Here's how the part is built. I have some questions about the finished solid (model axes, mm). Face numbers are marked on the shaded views. A direction names the side the tool comes from. Coordinates: 2 decimals unless noted, no trailing zeros. Write each loop counter-clockwise with the first axis right and the second up, starting at its lowest first coordinate (ties: lowest second). Pieces come first, ordered by that corner, then holes.
(1) Imagine slicing it at B-B, the plane x = 0. List the corners of the cut face in (y, z) for me, plus the area to 3 significant figures.
(2) Imagine slicing it at A-A, the plane y = 15.3. List the corners of the cut face in (x, z) for me.
(3) For pin 1 Ø1.5 at (x, y) = (39.99, 15.3) entering from -Z; pin 2 Ø3.5 at (x, y) = (34.5, -16) entering from +Z; pin 3 Ø1.6 at (y, z) = (12, -101.5) entering from -X; pin 4 Ø2.5 at (y, z) = (-16, -100.5) entering from -X, each with a flat end and sliding along its axis, tell me the tip position at first contact or that it passes through.
(4) Imagine slicing it at C-C, the plane x = 32. List the corners of the cut face in (y, z) for me, plus the area to 3 significant figures.
(5) Which directions (+Z, -Z, +X, -X, +Y, -Y) give clear straight access to the entire face, cutting with the end or side of a thin tool? Please do the marked faces 1, 2 and 3.
(6) Please list where these lines run through material, in increasing order: probe 1 along Y at (x, z) = (16, -88.25); probe 2 along Z at (x, y) = (38.5, -15.5); probe 3 along Z at (x, y) = (42, 12.5).
(7) Imagine slicing it at D-D, the plane y = -8. List the corners of the cut face in (x, z) for me, plus the area to 3 significant figures.
```python
from build123d import *

# Parameters (mm, degrees)
SKETCH_1_R          = 1.6
EXTRUDE_1_DEPTH     = 3
SKETCH_2_R          = 3.1
CUT_EXTRUDE_1_DEPTH = 2
FILLET_1_R          = 0.2
SKETCH_4_W          = 20
SKETCH_4_H          = 3.3
EXTRUDE_2_DEPTH     = 37
FILLET_2_R          = 2
SKETCH_5_R          = 1.25
CUT_EXTRUDE_2_DEPTH = 3.3


with BuildPart() as part:
    # Эскиз1 → Бобышка-Вытянуть1 (new body)
    with BuildSketch(Plane(origin=(0, -18, 0), x_dir=(1, 0, 0), z_dir=(0, 1, 0))):
        with BuildLine():
            Line((9.520833333, 86.731463811), (-1.458333333, 90.079283893))
            ThreePointArc((-1.458333333, 90.079283893), (-5, 94.861884011), (-1.458333333, 99.644484129))
            Line((-1.458333333, 99.644484129), (6.608333333, 102.104210763))
            ThreePointArc((6.608333333, 102.104210763), (7.495119036, 101.951328303), (7.9, 101.14769074))
            Line((7.9, 101.14769074), (7.9, 94.861884011))
            ThreePointArc((7.9, 94.861884011), (12, 90.761884011), (16.1, 94.861884011))
            Line((16.1, 94.861884011), (16.1, 102.361884011))
            ThreePointArc((16.1, 102.361884011), (16.392893219, 103.068990793), (17.1, 103.361884011))
            Line((17.1, 103.361884011), (44.988630488, 103.361884011))
            Line((44.988630488, 103.361884011), (44.988630488, 94.861884011))
            Line((44.988630488, 94.861884011), (29, 94.861884011))
            ThreePointArc((29, 94.861884011), (28.018187817, 91.886288833), (25.458333333, 90.079283893))
            Line((25.458333333, 90.079283893), (14.479166667, 86.731463811))
            ThreePointArc((14.479166667, 86.731463811), (12, 86.361884011), (9.520833333, 86.731463811))
        make_face()
        with Locations(Location((24, 94.861884011, 0), (0, 0, 270))):
            Circle(SKETCH_1_R, mode=Mode.SUBTRACT)
        with Locations(Location((0, 94.861884011, 0), (0, 0, 270))):
            Circle(SKETCH_1_R, mode=Mode.SUBTRACT)
    extrude(amount=EXTRUDE_1_DEPTH)

    # Эскиз2 → Вырез-Вытянуть1 (cut)
    with BuildSketch(Plane(origin=(0, -15, 0), x_dir=(1, 0, 0), z_dir=(0, 1, 0))):
        with Locations(Location((0, 94.861884011, 0), (0, 0, 270))):
            Circle(SKETCH_2_R)
        with Locations(Location((24, 94.861884011, 0), (0, 0, 270))):
            Circle(SKETCH_2_R)
    extrude(amount=-CUT_EXTRUDE_1_DEPTH, mode=Mode.SUBTRACT)

    # Скругление1
    fillet_1_edges = [part.edges().sort_by_distance(p)[0] for p in [
        (0, -17, -97.961884011),
        (24, -17, -97.961884011),
    ]]
    fillet(fillet_1_edges, radius=FILLET_1_R)

    # Эскиз4 → Бобышка-Вытянуть2 (add)
    with BuildSketch(Plane(origin=(0, -15, 0), x_dir=(1, 0, 0), z_dir=(0, 1, 0))):
        with Locations((34.988630488, 101.711884011)):
            Rectangle(SKETCH_4_W, SKETCH_4_H)
    extrude(amount=EXTRUDE_2_DEPTH)

    # Скругление2
    fillet_2_edges = [part.edges().sort_by_distance(p)[0] for p in [
        (44.988630488, 2, -103.361884011),
        (44.988630488, -16.5, -94.861884011),
        (29, -16.5, -94.861884011),
        (34.988630488, -15, -100.061884011),
    ]]
    fillet(fillet_2_edges, radius=FILLET_2_R)

    # Эскиз5 → Вырез-Вытянуть2 (cut)
    with BuildSketch(Plane.XY.offset(-100.061884011)):
        with Locations((39.988630488, 15.3)):
            Circle(SKETCH_5_R)
        with Locations((29.988630488, 15.3)):
            Circle(SKETCH_5_R)
    extrude(amount=-CUT_EXTRUDE_2_DEPTH, mode=Mode.SUBTRACT)


solid = part.part
```
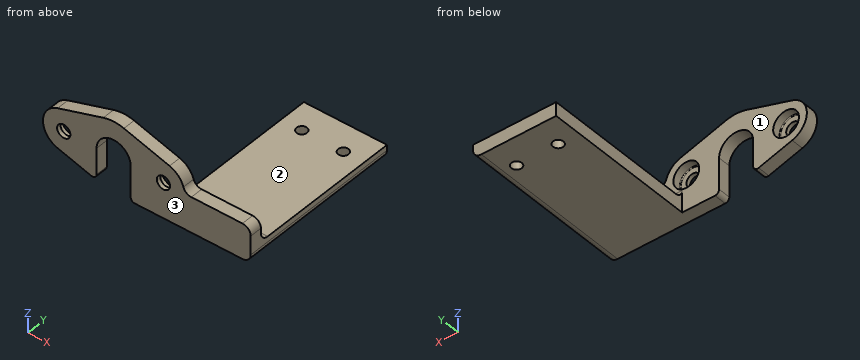
Recorded:
1. outline: (-18, -100.09) - (-15, -100.09) - (-15, -97.96) - (-16.8, -97.96) arc R0.2 cw to (-17, -97.76) - (-17, -96.46) - (-18, -96.46) - close; (-18, -93.26) - (-17, -93.26) - (-17, -91.96) arc R0.2 cw to (-16.8, -91.76) - (-15, -91.76) - (-15, -89.63) - (-18, -89.63) - close
1. area: 15.8 mm2
2. outline: (24.99, -103.36) - (28.74, -103.36) - (28.74, -100.06) - (24.99, -100.06) - close; (31.24, -103.36) - (38.74, -103.36) - (38.74, -100.06) - (31.24, -100.06) - close; (41.24, -103.36) - (42.99, -103.36) arc R2 ccw to (44.99, -101.36) - (44.99, -100.06) - (41.24, -100.06) - close
3. pin 1: passes through
3. pin 2: stops at z = -94.86
3. pin 3: stops at x = 24.99
3. pin 4: stops at x = -2.4
4. outline: (-18, -103.36) - (22, -103.36) - (22, -100.06) - (-13, -100.06) arc R2 cw to (-15, -98.06) - (-15, -94.86) - (-18, -94.86) - close
4. area: 148 mm2
5. face 1: +Z, -X, +Y
5. face 2: +Z, +X, -X, +Y
5. face 3: +Z, -Z, +X, -X, -Y
6. probe 1: y = -18 to -15
6. probe 2: z = -103.36 to -94.86
6. probe 3: z = -103.36 to -100.06
7. outline: (24.99, -103.36) - (42.99, -103.36) arc R2 ccw to (44.99, -101.36) - (44.99, -100.06) - (24.99, -100.06) - close
7. area: 65.1 mm2
